The drawing under review shows one solid part. Ordinate dimensions are in mm from its lowest x, y, z. A direction names the side the tool comes from. Give positions to 0.01 mm unless a question says otherwise; leave off trailing zeros. Loops run counter-clockwise (first coordinate to the right, second up) from the corner with the lowest first, then second, coordinate; pieces in that order, holes last. Notation, with made-up numbers: M 66.25,41.25 L 103.25,41.25 A23 cw 103.25,70.25 Z; hole C 57,62.25 d3. An arc over 180 degrees is marked long. One line per item, written item: value. Start each with the question number.
Q1. For the marked faces 4 and 5, list the 3-axis set-ups (+Z, -Z, +X, -X, +Y, -Y) from which the entire face can be reached by the end or side of a thin tool; tool diameter is ignored.
Q2. To check wall thickness, follow line 1 along Y through (x, z) = (6.5, 6.25); line 2 along X through (y, z) = (15, 5); line 3 along Z through (x, y) = (6.5, 3). State the ranges of each line that lie inside material, in increasing order. Write a range as from..to.
Q3. We need section C-C on z = 4.25. Write out the cut boundary in (x, y).
Q4. We need section D-D on x = 22. Write out the cut boundary in (y, z).
Q5. We need section B-B on x = 6.5. Write out the cut boundary in (y, z), plus the area to 3 significant figures.
Q6. Mouldability with a two-part tool opening along X and no side actions: class the marked faces 1, 2 and 3 as released by +X, released by -X, zero draft, split by the parting line, or undercut.
Q7. For pin 1 (1.6 mm diameter, centred on x = 9, z = 0.5, fed in from -Y); pin 2 (3 mm diameter, centred on x = 6.5, y = 4.5, fed in from -Z); pin 3 (0.9 mm diameter, centred on x = 27.5, z = 5.5, fed in from +Y); pin 4 (1.8 mm diameter, centred on x = 6.5, y = 12.5, fed in from +Z), all flat-tipped, find the tip position at first contact; note any pin that passes through.
Q8. We need section A-A on y = 4.5. Write out the cut boundary in (x, z), plus the area to 4 significant figures.
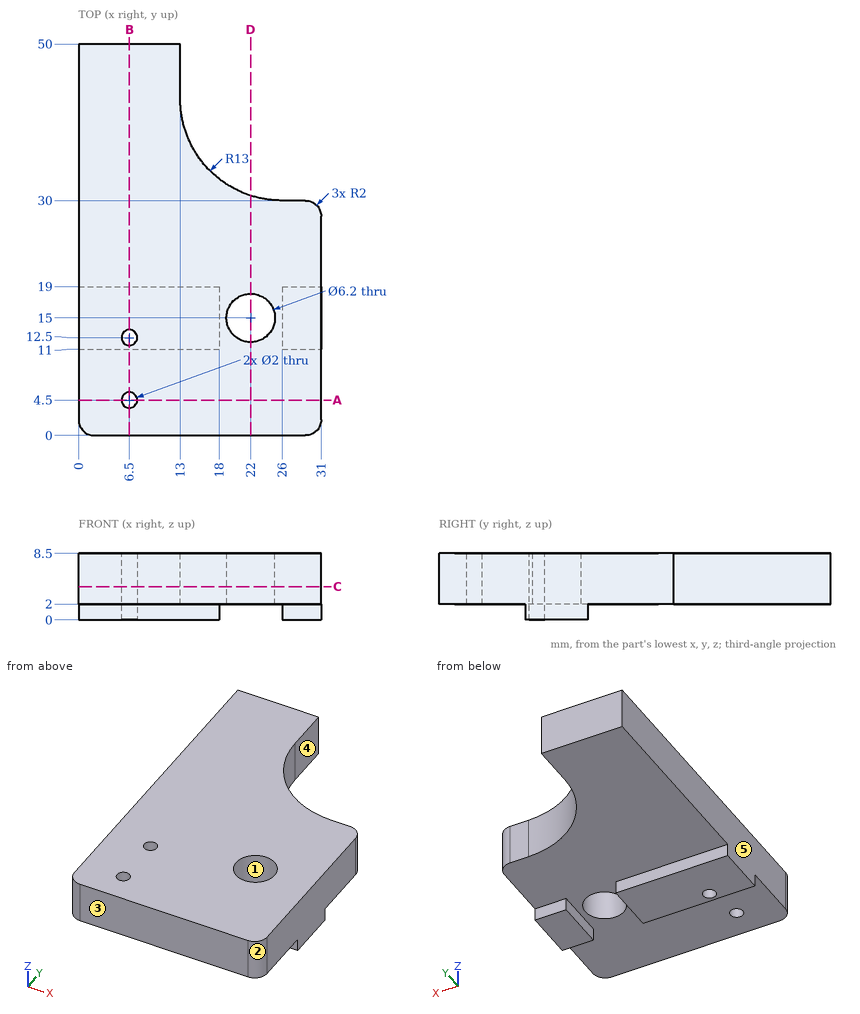
Solved:
1. face 4: +Z, -Z, +X, +Y
1. face 5: +Z, -Z, -X, +Y, -Y
2. line 1: 0..3.5, 5.5..11.5, 13.5..50
2. line 2: 0..18.9, 25.1..31
2. line 3: 2..8.5
3. outline: M 0,2 A2 ccw 2,0 L 29,0 A2 ccw 31,2 L 31,28 A2 ccw 29,30 L 26,30 A13 cw 13,43 L 13,50 L 0,50 Z; hole C 6.5,4.5 d2; hole C 6.5,12.5 d2; hole C 22,15 d6.2
4. outline: M 0,2 L 11.9,2 L 11.9,8.5 L 0,8.5 Z; M 18.1,2 L 30.63,2 L 30.63,8.5 L 18.1,8.5 Z
5. outline: M 0,2 L 3.5,2 L 3.5,8.5 L 0,8.5 Z; M 5.5,2 L 11,2 L 11,0 L 11.5,0 L 11.5,8.5 L 5.5,8.5 Z; M 13.5,0 L 19,0 L 19,2 L 50,2 L 50,8.5 L 13.5,8.5 Z
5. area: 311 mm2
6. face 1: undercut
6. face 2: released by +X
6. face 3: zero draft
7. pin 1: y = 11
7. pin 2: z = 2
7. pin 3: y = 30
7. pin 4: through
8. outline: M 0,2 L 5.5,2 L 5.5,8.5 L 0,8.5 Z; M 7.5,2 L 31,2 L 31,8.5 L 7.5,8.5 Z
8. area: 188.5 mm2
